from build123d import *

# Parameters (mm, degrees)
SKETCH_R            = 1.4
SKETCH_W            = 29.4
SKETCH_H            = 15.4
SKETCH_W_2          = 38.5
SKETCH_H_2          = 28
SKETCH_W_3          = 11.1
SKETCH_H_3          = 73.8
SKETCH_W_4          = 10.132
SKETCH_W_5          = 69.6
SKETCH_H_4          = 33.8
SKETCH_H_5          = 30
PAD_DEPTH           = 3
SKETCH001_R         = 3.7
SKETCH001_R_2       = 1.025
PAD001_DEPTH        = 11
SKETCH002_W         = 35
SKETCH002_H         = 5
PAD002_DEPTH        = 32
PAD002_DEPTH_BACK   = 3
HOLE_D              = 3.4
HOLE_DEPTH          = 25
HOLE_CSINK_D        = 8
HOLE_CSINK_ANGLE    = 90
PAD003_DEPTH        = 2.5
HOLE002_D           = 1.71
HOLE002_DEPTH       = 25
HOLE002_CSINK_D     = 3.5
HOLE002_CSINK_ANGLE = 90


with BuildPart() as part:
    # Sketch → Pad (new body)
    with BuildSketch(Plane.XZ):
        Polygon((-54.8, 252.6), (-54.8, 16), (-54.8, 0), (54.8, 0), (54.8, 16), (54.8, 252.6), align=None)
        with Locations((-24.13, 243.52)):
            Circle(SKETCH_R, mode=Mode.SUBTRACT)
        with Locations((46.99, 243.52)):
            Circle(SKETCH_R, mode=Mode.SUBTRACT)
        with Locations((-46.99, 45.5)):
            Circle(SKETCH_R, mode=Mode.SUBTRACT)
        with Locations((46.99, 45.5)):
            Circle(SKETCH_R, mode=Mode.SUBTRACT)
        with Locations((-14.668, 124.14)):
            Circle(SKETCH_R, mode=Mode.SUBTRACT)
        with Locations((-46.99, 180.78)):
            Circle(SKETCH_R, mode=Mode.SUBTRACT)
        with Locations((46.99, 164.78)):
            Circle(SKETCH_R, mode=Mode.SUBTRACT)
        with Locations((17.1, 154.5)):
            Rectangle(SKETCH_W, SKETCH_H, mode=Mode.SUBTRACT)
        with Locations((15.55, 120.8)):
            Rectangle(SKETCH_W_2, SKETCH_H_2, mode=Mode.SUBTRACT)
        with Locations((17.1, 229.9)):
            Rectangle(SKETCH_W, SKETCH_H, mode=Mode.SUBTRACT)
        with Locations((15.55, 196.2)):
            Rectangle(SKETCH_W_2, SKETCH_H_2, mode=Mode.SUBTRACT)
        with Locations((-29.25, 191.7)):
            Rectangle(SKETCH_W_3, SKETCH_H_3, mode=Mode.SUBTRACT)
        with Locations((-29.734, 120.8)):
            Rectangle(SKETCH_W_4, SKETCH_H_2, mode=Mode.SUBTRACT)
        with Locations((0, 77.9)):
            Rectangle(SKETCH_W_5, SKETCH_H_4, mode=Mode.SUBTRACT)
        with Locations((0, 31)):
            Rectangle(SKETCH_W_5, SKETCH_H_5, mode=Mode.SUBTRACT)
    extrude(amount=-PAD_DEPTH)

    # Sketch001 → Pad001 (join)
    with BuildSketch(Plane.XZ):
        with Locations((-24.13, 243.52)):
            Circle(SKETCH001_R)
        with Locations((-24.13, 243.52)):
            Circle(SKETCH001_R_2, mode=Mode.SUBTRACT)
        with Locations((46.99, 243.52)):
            Circle(SKETCH001_R)
        with Locations((46.99, 243.52)):
            Circle(SKETCH001_R_2, mode=Mode.SUBTRACT)
        with Locations((-46.99, 180.78)):
            Circle(SKETCH001_R)
        with Locations((-46.99, 180.78)):
            Circle(SKETCH001_R_2, mode=Mode.SUBTRACT)
        with Locations((46.99, 164.78)):
            Circle(SKETCH001_R)
        with Locations((46.99, 164.78)):
            Circle(SKETCH001_R_2, mode=Mode.SUBTRACT)
        with Locations((-14.668, 124.14)):
            Circle(SKETCH001_R)
        with Locations((-14.668, 124.14)):
            Circle(SKETCH001_R_2, mode=Mode.SUBTRACT)
        with Locations((-46.99, 45.5)):
            Circle(SKETCH001_R)
        with Locations((-46.99, 45.5)):
            Circle(SKETCH001_R_2, mode=Mode.SUBTRACT)
        with Locations((46.99, 45.5)):
            Circle(SKETCH001_R)
        with Locations((46.99, 45.5)):
            Circle(SKETCH001_R_2, mode=Mode.SUBTRACT)
    extrude(amount=PAD001_DEPTH)

    # Sketch002 → Pad002 (join, two sides)
    with BuildSketch(Plane.XZ) as pad002_sk:
        with Locations((-37.3, -2.5)):
            Rectangle(SKETCH002_W, SKETCH002_H)
        with Locations((37.3, -2.5)):
            Rectangle(SKETCH002_W, SKETCH002_H)
    extrude(amount=PAD002_DEPTH)
    extrude(pad002_sk.sketch, amount=-PAD002_DEPTH_BACK)

    # Hole
    with Locations(Plane.XY):
        with Locations((-37.3, -16), (37.3, -16)):
            CounterSinkHole(HOLE_D / 2, HOLE_CSINK_D / 2, depth=HOLE_DEPTH, counter_sink_angle=HOLE_CSINK_ANGLE)

    # Sketch004 (on DatumPlane) → Pad003 (join)
    with BuildSketch(Plane.YZ.offset(54.8)):
        Polygon((-25.8, -5), (3, -5), (3, 28), align=None)
        Polygon((-10.8, 1), (-3, 13), (-3, 1), align=None, mode=Mode.SUBTRACT)
    pad003 = extrude(amount=PAD003_DEPTH)

    # Mirrored: Pad003 across YZ
    add(pad003.mirror(Plane.YZ))

    # Hole002
    with Locations(Plane.XZ):
        with Locations((44.8, 157), (-44.8, 135), (44.8, 135), (-44.8, 112), (-44.8, 94), (44.8, 112), (44.8, 94), (-44.8, 30), (44.8, 30), (-44.8, 157), (-44.8, 230), (44.8, 230)):
            CounterSinkHole(HOLE002_D / 2, HOLE002_CSINK_D / 2, depth=HOLE002_DEPTH, counter_sink_angle=HOLE002_CSINK_ANGLE)


with BuildPart() as part_1:
    # Body placement: moved
    add(part.part.moved(Location((0.2, -1, 0))))


solid = part_1.part
Geometry: final body of the model. Coordinates: model frame, mm. A direction names the side the tool comes from. Give positions to 0.01 mm unless a question says otherwise; leave off trailing zeros. Order: outer loops, then holes, each group sorted by start corner. A loop starts at its lowest first (then second) coordinate and runs counter-clockwise, first axis right, second up. Notation, with made-up numbers: (29, 61) -> (58, 61) arc R29 cw to (58, 81) -> close; hole circle Ø10 at (19, 45). An arc over 180 degrees is marked (long way). Put each result on its own line as item: value.
Q1. Section D-D, the plane x = 13. Return loops of the section in (y, z).
Here are the results:
outline: (-1, 0) -> (2, 0) -> (2, 16) -> (-1, 16) -> close; (-1, 46) -> (2, 46) -> (2, 61) -> (-1, 61) -> close; (-1, 94.8) -> (2, 94.8) -> (2, 106.8) -> (-1, 106.8) -> close; (-1, 134.8) -> (2, 134.8) -> (2, 146.8) -> (-1, 146.8) -> close; (-1, 162.2) -> (2, 162.2) -> (2, 182.2) -> (-1, 182.2) -> close; (-1, 210.2) -> (2, 210.2) -> (2, 222.2) -> (-1, 222.2) -> close; (-1, 237.6) -> (2, 237.6) -> (2, 252.6) -> (-1, 252.6) -> close
Q2. Draft query along X for faces 1 (the face through (-54.6, -29, -3)), 2 (the face through (-47.27, -6.42, 49.17)), 3 (the face through (55, -29, -3)), 4 (the face through (56.23, -12.2, 11.73)). Return one class per face: released by +X, released by -X, zero draft, split by the parting line, or undercut.
Here are the results:
face 1: released by -X
face 2: undercut
face 3: released by +X
face 4: zero draft
Q3. Pin query (flat end, axial travel): pin 1 (1.5 mm diameter, centred on y = 0.5, z = 115.5, fed in from -X); pin 2 (3.5 mm diameter, centred on x = 48.5, z = 242, fed in from -Y); pin 3 (2.5 mm diameter, centred on x = 45, z = 157, fed in from +Y); pin 4 (2 mm diameter, centred on x = -37.1, y = -17, fed in from +Z) (1 decimal). Return the tip coordinate at first contact, or that it passes through.
Here are the results:
pin 1: stops at x = -54.6
pin 2: stops at y = -12
pin 3: stops at y = 2
pin 4: passes through
Q4. Material intervals for L1, parallel to X at y = 0, z = 112 (3 decimals); L2, parallel to X at y = 1.3, z = 135 (3 decimals); L3, parallel to Z at x = 26, y = -26.5, sorted ascending.
Here are the results:
L1: x = -54.6 to -45.455, -43.745 to -34.6, -24.468 to -3.5, 35 to 44.145, 45.855 to 55
L2: x = -54.6 to -45.455, -43.745 to 44.145, 45.855 to 55
L3: z = -5 to 0
Q5. Section B-B, the plane y = -7. Count the separate pieces of the cut face and the enclosed holes in it, then the cut area to 3 significant figures.
Here are the results:
separate pieces: 11
enclosed holes: 7
area: 704 mm^2
Q6. Section C-C, the plane z = 65. Return loops of the section in (x, y).
Here are the results:
outline: (-54.6, -1) -> (-34.6, -1) -> (-34.6, 2) -> (-54.6, 2) -> close; (35, -1) -> (55, -1) -> (55, 2) -> (35, 2) -> close
Q7. Section A-A, the plane x = -30. Return loops of the section in (y, z).
Here are the results:
outline: (-33, -5) -> (2, -5) -> (2, 16) -> (-1, 16) -> (-1, 0) -> (-33, 0) -> close; (-1, 46) -> (2, 46) -> (2, 61) -> (-1, 61) -> close; (-1, 94.8) -> (2, 94.8) -> (2, 106.8) -> (-1, 106.8) -> close; (-1, 134.8) -> (2, 134.8) -> (2, 154.8) -> (-1, 154.8) -> close; (-1, 228.6) -> (2, 228.6) -> (2, 252.6) -> (-1, 252.6) -> close
Q8. Reachability of faces 5 (the face through (-26.66, -6.42, 246.02)), 6 (the face through (-46, -12, 46.4)), 7 (the face through (-54.6, -9, 10)) from +Z, -Z, +X, -X, +Y, -Y: full face, straight path, thin tool, end or side. Return the list, or none.
Here are the results:
face 5: -Y
face 6: +Z, +X, -X, -Y
face 7: +Z, -Y
